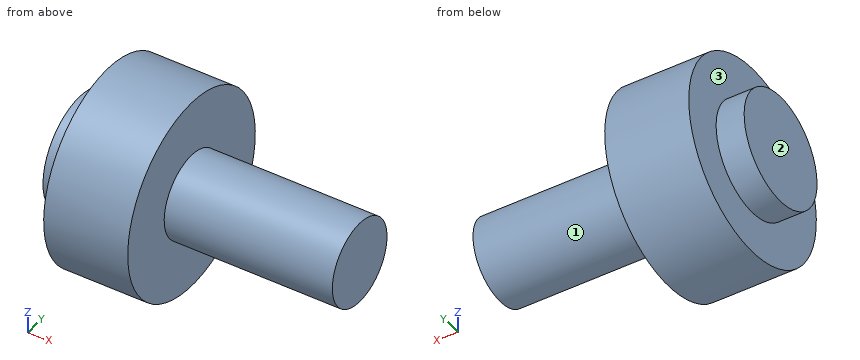
```python
from build123d import *

# Parameters (mm, degrees)
SKETCH_2_R          = 5
CUT_EXTRUDE_1_DEPTH = 20


with BuildPart() as part:
    # Эскиз1 → Повернуть1 (revolve)
    with BuildSketch(Plane.XY, mode=Mode.PRIVATE) as revolve_1_sk:
        Polygon((0, 0), (100, 0), (100, 15), (40, 15), (40, 35), (10, 35), (10, 20), (0, 20), align=None)
    revolve(revolve_1_sk.sketch.rotate(Axis((0, 0, 0), (1, 0, 0)), 90), axis=Axis((0, 0, 0), (1, 0, 0)))

    # Эскиз2 → Вырез-Вытянуть1 (cut)
    with BuildSketch(Plane(origin=(25, 0, 0), x_dir=(0, 0, -1), z_dir=(1, 0, 0))):
        Circle(SKETCH_2_R)
    extrude(amount=CUT_EXTRUDE_1_DEPTH, mode=Mode.SUBTRACT)


solid = part.part
```
Geometry: final body of the model. Coordinates: model frame, mm. Face numbers are marked on the shaded views. A direction names the side the tool comes from. Give positions to 0.01 mm unless a question says otherwise; leave off trailing zeros. Write each loop counter-clockwise with the first axis right and the second up, starting at its lowest first coordinate (ties: lowest second). Pieces come first, ordered by that corner, then holes.
1. Pin query (flat end, axial travel): P1, Ø12, axis at x = 33.5, z = 15, coming from the -Y side; P2, Ø2, axis at y = 12.5, z = 15, coming from the -X side; P3, Ø1.5, axis at x = 24, y = -24, coming from the -Z side; P4, Ø1, axis at x = 31, y = -9, coming from the +Z side. Return the tip coordinate at first contact, or that it passes through.
2. Section query A-A, the plane y = 0. Return loops of the section in (x, z).
3. Reachability of the marked faces 1, 2 and 3 from +Z, -Z, +X, -X, +Y, -Y: full face, straight path, thin tool, end or side. Return the list, or none.
4. Section query C-C, the plane x = 56. Return loops of the section in (y, z), then the cut area to 3 significant figures.
5. Line query: probe 1 along Y at (x, z) = (38, 0); probe 2 along Z at (x, y) = (35, -0.5); probe 3 along X at (y, z) = (-1, -26). Output: solid intervals per line, ascending.
6. Section query D-D, the plane z = 8. Return loops of the section in (x, y).
Computed:
1. P1: stops at y = -33.82
1. P2: stops at x = 0
1. P3: stops at z = -26.16
1. P4: stops at z = 33.95
2. outline: (0, -20) - (10, -20) - (10, -35) - (40, -35) - (40, -15) - (100, -15) - (100, 15) - (40, 15) - (40, 35) - (10, 35) - (10, 20) - (0, 20) - close; hole (25, -5) - (45, -5) - (45, 5) - (25, 5) - close
3. face 1: +X
3. face 2: +Z, -Z, -X, +Y, -Y
3. face 3: -X
4. outline: circle Ø30 at (0, 0)
4. area: 707 mm2
5. probe 1: y = -35 to -5, 5 to 35
5. probe 2: z = -35 to -4.97, 4.97 to 35
5. probe 3: x = 10 to 40
6. outline: (0, -18.33) - (10, -18.33) - (10, -34.07) - (40, -34.07) - (40, -12.69) - (100, -12.69) - (100, 12.69) - (40, 12.69) - (40, 34.07) - (10, 34.07) - (10, 18.33) - (0, 18.33) - close
